Verification items for this drawing (mm, ordinates from the low corner). A direction names the side the tool comes from. Round coordinates to 2 decimals unless told otherwise and drop trailing zeros. Order: outer loops, then holes, each group sorted by start corner. A loop starts at its lowest first (then second) coordinate and runs counter-clockwise, first axis right, second up.
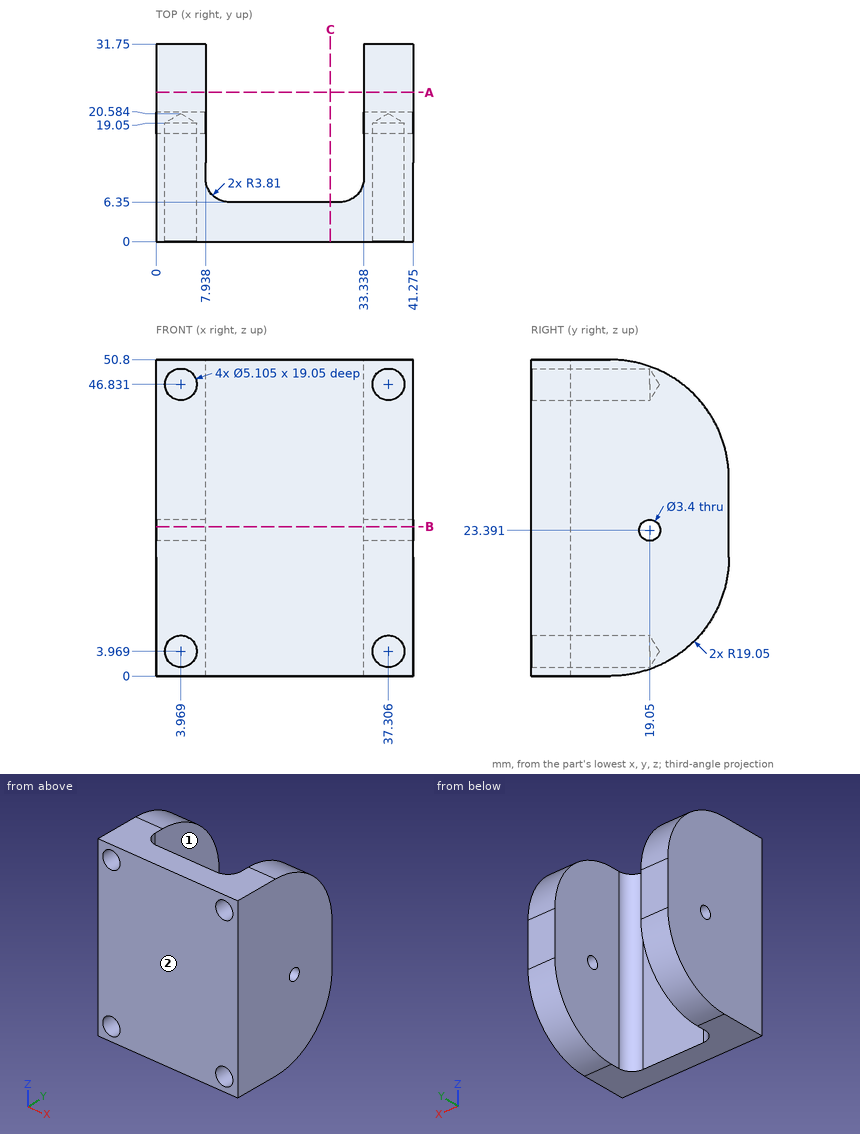
Item 1: Sectioned sample at A-A (y = 24). Record the cut outline in (x, z) (1 decimal).
Answer:
outline: (0, 3.7) - (7.9, 3.7) - (7.9, 47.1) - (0, 47.1) - close; (33.3, 3.7) - (41.3, 3.7) - (41.3, 47.1) - (33.3, 47.1) - close
Item 2: Sectioned sample at B-B (z = 24). State how many separate pieces and enclosed holes the cut face has, and give its area (3 significant figures).
Answer:
separate pieces: 3
enclosed holes: 0
area: 621 mm2
Item 3: Access from +Z, -Z, +X, -X, +Y, -Y to the whole of each face (thin tool, end or side, straight path). Record for the marked faces 1 and 2.
Answer:
face 1: +Z, -Z, +Y
face 2: +Z, -Z, +X, -X, -Y
Item 4: Go/stop test with flat-tipped pins: P1, Ø3, axis at x = 8, z = 12, coming from the +Y side; P2, Ø3, axis at x = 5, y = 22, coming from the +Z side; P3, Ø4.5, axis at x = 3.97, z = 46.83, coming from the -Y side; P4, Ø3, axis at y = 19.05, z = 23.39, coming from the +X side. Record where each tip stops, or that it passes through.
Answer:
P1: stops at y = 30.92
P2: stops at z = 49.13
P3: stops at y = 19.23
P4: passes through
Item 5: Sectioned sample at C-C (x = 28). Record the cut outline in (y, z).
Answer:
outline: (0, 0) - (6.35, 0) - (6.35, 50.8) - (0, 50.8) - close
Item 6: Scan lines: line 1 along X through (y, z) = (26.5, 33) (1 decimal); line 2 along Z through (x, y) = (35, 19) (1 decimal); line 3 along X through (y, z) = (14, 46) (1 decimal). Record each from-to range of solid material in increasing order.
Answer:
line 1: x = 0 to 7.9, 33.3 to 41.3
line 2: z = 1.1 to 2.9, 5.1 to 21.7, 25.1 to 45.7, 47.9 to 49.7
line 3: x = 0 to 1.6, 6.4 to 7.9, 33.3 to 34.9, 39.7 to 41.3
